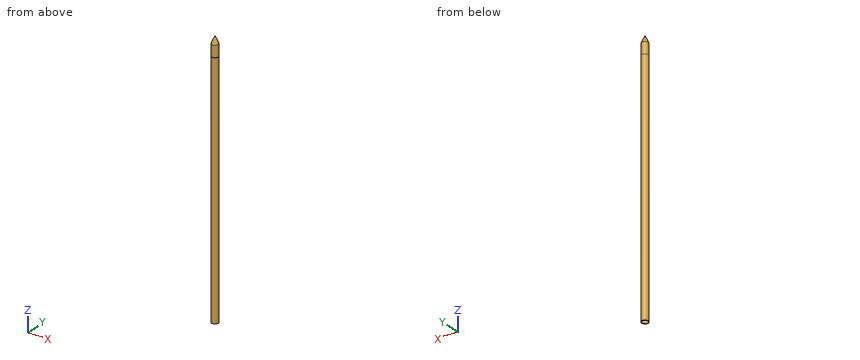
Autodesk Inventor part; units mm, degrees
ref_plane "YZ Plane" through (0, 0, 0) normal (1, 0, 0) x (0, 1, 0)
ref_plane "XZ Plane" through (0, 0, 0) normal (0, 1, 0) x (-1, 0, 0)
ref_plane "XY Plane" through (0, 0, 0) normal (0, 0, 1) x (1, 0, 0)
sketch "草圖1" plane through (0, 0, 0) normal (0, 1, 0) x (-1, 0, 0)
  line L0 (0, 0) -> (0, -115)
  line L1 (0, -115) -> (1.5, -115)
  line L2 (1.5, -115) -> (1.5, -8)
  line L3 (1.5, -8) -> (1.5, -8.1)
  line L4 (1.5, -8) -> (1.4, -8)
  line L5 (1.4, -8) -> (1.4, -3)
  line L6 (0, 0) -> (0.0831, 0) construction
  line L7 (0.0831, 0) -> (0.4369, -0.6984) construction
  line L8 (0.4369, -0.6984) -> (0.929, -1.7279) construction
  line L9 (0.929, -1.7279) -> (1.4, -2.7133) construction
  line L10 (1.4, -2.7133) -> (1.4, -3) construction
  spline S0 degree 4 poles (0, 0) (0.0831, 0) (0.4369, -0.6984) (0.929, -1.7279) (1.4, -2.7133) (1.4, -3) knots 0 0 0 0 0 1 2 2 2 2 2
  line L11 (1.5, -8) -> (1.5, -21)
  arc A0 (1.5836, -22.9983) -> (1.5, -21) centre (1.5558, -21.9985) ccw
  dimension "d0" = 115
  dimension "d1" = 1.5
  dimension "d2" = 107
  dimension "d4" = 0.1
  dimension "d5" = 5
  dimension "d8" = 13
  dimension "d9" = 2
  dimension "d10" = 1.0001
revolve "迴轉1" add sketch "草圖1" angle 360 about axis through (0, 0, 0) along (0, 0, -1)
sketch "草圖2" plane through (0, 0, -115) normal (0, 0, -1) x (-1, 0, 0)
  point P0 (0, 0)
  point P1 (0, 0)
hole "孔1" at (0, 0, -115) direction (0, 0, 1) diameter 2.5 depth 105 tip angle 118
properties part number "筆芯"
Source: CAD feature listing. Evaluate the final solid. Frame: model axes, mm. Give positions to 0.01 mm unless a question says otherwise; leave off trailing zeros. Loops run counter-clockwise (first coordinate to the right, second up) from the corner with the lowest first, then second, coordinate; pieces in that order, holes last. Notation, with made-up numbers: (-30.5, 30) -> (-6.5, 30) arc R25 ccw to (-6.5, 43) -> close; hole circle Ø2 at (-27.5, 27). An arc over 180 degrees is marked (long way). Put each result on its own line as item: value. Start each with the question number.
1) Cut plane A-A (z = -88.5). Return loops of the section in (x, y), then the cut area to 3 significant figures.
2) Material intervals for probe 1 along Y at (x, z) = (0, -54); probe 2 along X at (y, z) = (0.15, -77.5); probe 3 along Y at (x, z) = (-0.6, -4.5), sorted ascending.
3) Contact query for flat-ended pins moving along their axis: P1, Ø1.5, axis at x = 1, z = -90, coming from the -Y side; P2, Ø1.5, axis at x = 0, y = 0, coming from the -Z side. Output: stop coordinate, or through.
Results are:
1. outline: circle Ø3 at (0, 0); hole circle Ø2.5 at (0, 0)
1. area: 2.16 mm2
2. probe 1: y = -1.5 to -1.25, 1.25 to 1.5
2. probe 2: x = -1.49 to -1.24, 1.24 to 1.49
2. probe 3: y = -1.26 to 1.26
3. P1: stops at y = -1.48
3. P2: stops at z = -9.7
